```python
from build123d import *

# Parameters (mm, degrees)
F0_R     = 100
F0_R_2   = 52.5
F1_DEPTH = 60
F3_W     = 230
F3_H     = 250
F4_DEPTH = 15
F2_R     = 9.3755397544
F5_DEPTH = 75.001
F6_R     = 38.5
F7_DEPTH = 15.001
F9_D     = 8.5
F9_DEPTH = 16.5
F9_TIP   = 2.5536576309
F10_R    = 5


with BuildPart() as f1:
    # F0 (on Front) → F1 (new body)
    with BuildSketch(Plane.XZ):
        Circle(F0_R)
        Circle(F0_R_2, mode=Mode.SUBTRACT)
    extrude(amount=F1_DEPTH)

    # F3 (on face) → F4 (join)
    with BuildSketch(Plane(origin=(0, 0, 0), x_dir=(-1, 0, 0), z_dir=(0, 1, 0))):
        Rectangle(F3_W, F3_H)
    extrude(amount=F4_DEPTH)

    # F2 (on face) → F5 (cut, through all)
    with BuildSketch(Plane.XZ.offset(60)):
        with Locations((-59.8148740828, 46.2548695505)):
            Circle(F2_R)
        with Locations((-69.9653291208, -28.6737657046)):
            Circle(F2_R)
        with Locations((-10.150455038, -74.9286352551)):
            Circle(F2_R)
        with Locations((59.8148740828, -46.2548695505)):
            Circle(F2_R)
        with Locations((69.9653291208, 28.6737657046)):
            Circle(F2_R)
        with Locations((10.150455038, 74.9286352551)):
            Circle(F2_R)
    extrude(amount=-F5_DEPTH, mode=Mode.SUBTRACT)

    # F6 (on face) → F7 (cut, through all)
    with BuildSketch(Plane.XZ):
        Circle(F6_R)
    extrude(amount=-F7_DEPTH, mode=Mode.SUBTRACT)

    # F9
    with Locations(Plane.XZ.offset(60)):
        with Locations((-45.0271219015, -55.2673339844), (-25.3493542792, 66.6282984182), (70.3764761807, -11.3609644338)):
            Hole(F9_D / 2, depth=F9_DEPTH)
            with Locations((0, 0, -(F9_DEPTH + F9_TIP / 2))):  # 118° drill point
                Cone(0, F9_D / 2, F9_TIP, mode=Mode.SUBTRACT)

    # F10
    f10_edges = [f1.edges().sort_by_distance(p)[0] for p in [
        (0, 0, 125),
        (115, 0, 0),
        (0, 0, -125),
        (-115, 0, 0),
    ]]
    fillet(f10_edges, radius=F10_R)


solid = f1.part
```
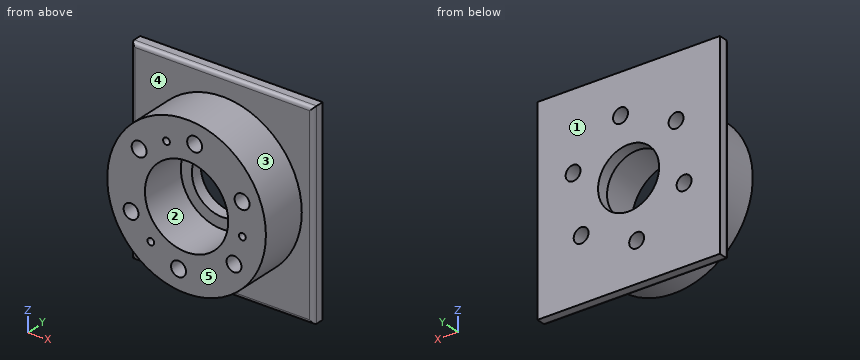
Read the model definition and answer for the solid it produces. Units are mm, in the model's axes. Face numbers are marked on the shaded views. A direction names the side the tool comes from. Round coordinates to 2 decimals unless told otherwise and drop trailing zeros. Write each loop counter-clockwise with the first axis right and the second up, starting at its lowest first coordinate (ties: lowest second). Pieces come first, ordered by that corner, then holes. Notation, with made-up numbers: M -33.75,8 L 16.25,8 A31 cw 16.25,43 Z; hole C 8.25,52 d1. An arc over 180 degrees is marked long. One line per item, written item: value.
Q1. Find section C-C on y = -54. Count the separate pieces of the cut face and the enclosed holes in it, plus the area to 3 significant figures.
Data:
separate pieces: 1
enclosed holes: 10
area: 20,900 mm2
Q2. Find section D-D on x = 47. Write down the section's boundary in (y, z), plus the area to 3 significant figures.
Data:
outline: M -60,-88.27 L 0,-88.27 L 0,-120 A5 ccw 5,-125 L 15,-125 L 15,125 L 5,125 A5 ccw 0,120 L 0,88.27 L -60,88.27 L -60,23.39 L 0,23.39 L 0,-23.39 L -60,-23.39 Z
area: 11,500 mm2
Q3. Find section A-A on z = 0. Write down the section's boundary in (x, y), plus the area to 3 significant figures.
Data:
outline: M -115,5 A5 ccw -110,0 L -100,0 L -100,-60 L -52.5,-60 L -52.5,0 L -38.5,0 L -38.5,15 L -115,15 Z; M 38.5,0 L 52.5,0 L 52.5,-60 L 100,-60 L 100,0 L 110,0 A5 ccw 115,5 L 115,15 L 38.5,15 Z
area: 7,980 mm2
Q4. Which of the six approach directions +Z, -Z, +X, -X, +Y, -Y give full straight-line access (tool end or side, diameter ignored) to the marked faces 4 and 5?
Data:
face 4: -Y
face 5: +Z, -Z, +X, -X, -Y
Q5. Straight lines are drawn through the part: line 1 (Z direction, x = 0, y = -47.5); line 2 (Z direction, x = -64, y = -3.5); line 3 (Z direction, x = -24.5, y = -47). For each, find the intervals that lie inside material, in ascending order. Write a range as [from, to].
Data:
line 1: [-100, -52.5], [52.5, 100]
line 2: [-76.84, -35.91], [-21.44, 37.87], [54.64, 76.84]
line 3: [-96.95, -46.43], [46.43, 62.46], [70.79, 96.95]
Q6. For a pull along Z with two mould halves and no side action, classify the marked faces 1, 2 and 3 as +Z half, -Z half, draft (parallel to the pull), parting line (faces both ways), or undercut.
Data:
face 1: draft
face 2: undercut
face 3: parting line
Q7. Flat-ended cylindrical pins translate along their axes: pin 1 Ø6 at (y, z) = (-48, -42.5) entering from +X; pin 2 Ø2 at (y, z) = (-37.5, -39) entering from -X; pin 3 Ø1 at (x, y) = (89, 0.5) entering from +Z. Find the tip coordinate at first contact, or state that the pin passes through.
Data:
pin 1: x = 91.87
pin 2: x = -92.5
pin 3: z = 123
Q8. Find section B-B on x = 24. Write down the section's boundary in (y, z), plus the area to 3 significant figures.
Data:
outline: M -60,-97.08 L 0,-97.08 L 0,-120 A5 ccw 5,-125 L 15,-125 L 15,-30.1 L 0,-30.1 L 0,-46.69 L -60,-46.69 Z; M -60,46.69 L 0,46.69 L 0,30.1 L 15,30.1 L 15,125 L 5,125 A5 ccw 0,120 L 0,97.08 L -60,97.08 Z
area: 8,880 mm2
